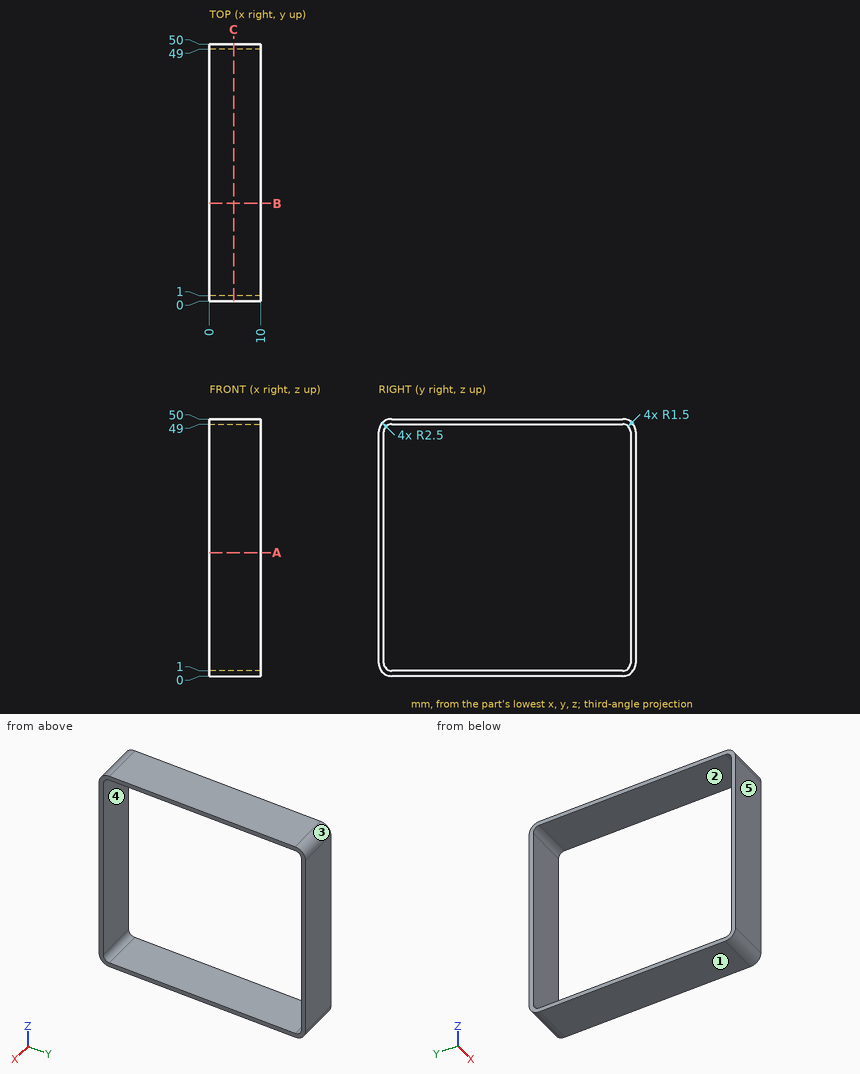
Here's the drawing with two shaded views (mm, measured from the low corner). I have some questions. A direction names the side the tool comes from. Give positions to 0.01 mm unless a question says otherwise; leave off trailing zeros. Write each loop counter-clockwise with the first axis right and the second up, starting at its lowest first coordinate (ties: lowest second). Pieces come first, ordered by that corner, then holes. Notation, with made-up numbers: (-2, 25) -> (3, 25) arc R16 ccw to (3, 54) -> close; hole circle Ø10 at (71.25, 16). An arc over 180 degrees is marked (long way). One line per item, written item: value.
Q1. Please list where this line runs through material, in increasing order: line 1 (Z direction, x = 0.75, y = 42.5). Write a range as [from, to].
Results found:
line 1: z = [0, 1], [49, 50]
Q2. We'd pull the mould along Y, two halves only. Please class the marked faces 3, 4 and 5: +Y half, -Y half, draft (parallel to the pull), parting line (faces both ways), or undercut.
Results found:
face 3: +Y half
face 4: undercut
face 5: -Y half
Q3. Imagine slicing it at C-C on x = 4.75. Please give me the cut outline in (y, z), and give its area (3 significant figures).
Results found:
outline: (0, 2.5) arc R2.5 ccw to (2.5, 0) -> (47.5, 0) arc R2.5 ccw to (50, 2.5) -> (50, 47.5) arc R2.5 ccw to (47.5, 50) -> (2.5, 50) arc R2.5 ccw to (0, 47.5) -> close; hole (1, 2.5) arc R1.5 ccw to (2.5, 1) -> (47.5, 1) arc R1.5 ccw to (49, 2.5) -> (49, 47.5) arc R1.5 ccw to (47.5, 49) -> (2.5, 49) arc R1.5 ccw to (1, 47.5) -> close
area: 193 mm^2
Q4. Which directions (+Z, -Z, +X, -X, +Y, -Y) give clear straight access to the entire face, cutting with the end or side of a thin tool? Please do the marked faces 1 and 2.
Results found:
face 1: -Z, +X, -X, +Y, -Y
face 2: +X, -X
Q5. Imagine slicing it at A-A on z = 24. Please give me the cut outline in (x, y).
Results found:
outline: (0, 0) -> (10, 0) -> (10, 1) -> (0, 1) -> close; (0, 49) -> (10, 49) -> (10, 50) -> (0, 50) -> close
